Part model, mm, in its own coordinate system. Coordinates: 2 decimals unless noted, no trailing zeros. Write each loop counter-clockwise with the first axis right and the second up, starting at its lowest first coordinate (ties: lowest second). Pieces come first, ordered by that corner, then holes. Notation, with made-up numbers: (-18.5, -39) -> (-3.5, -39) arc R32 cw to (-3.5, -7) -> close; hole circle Ø7 at (-8, -22.5). An arc over 180 degrees is marked (long way). One line per question, with ' | ' between items. Start each with the question number.
Item 1: Saw through at B-B (y = -3.25). List the corners of the cut face in (x, z).
Item 2: Saw through at D-D (z = 0.25). List the corners of the cut face in (x, y), and give its area (3 significant figures).
Item 3: Saw through at C-C (x = 6). List the corners of the cut face in (y, z).
Item 4: Pin check, flat tips, straight feed: pin 1 (4 mm diameter, centred on x = -7, y = 4.5, fed in from -Z); pin 2 (1 mm diameter, centred on y = -5, z = 0.5, fed in from +X); pin 3 (1 mm diameter, centred on x = -6.5, z = 1, fed in from -Y). Stop position of each tip, or through.
Item 5: Probe probe 1 along Z at (x, y) = (-5, 4.5); probe 2 along Y at (x, z) = (1.5, 0.4); probe 3 along Y at (x, z) = (-3.25, 0.35). List the from-to ranges inside material, lowest first. Write a range as [from, to].
Item 6: Saw through at A-A (z = 1.75). List the corners of the cut face in (x, y).
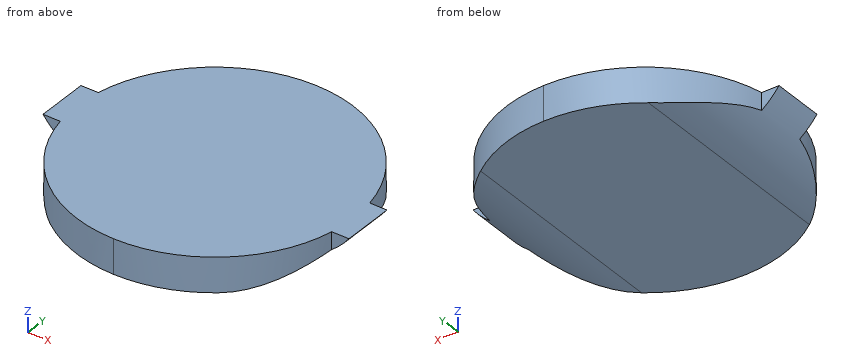
from build123d import *

# Parameters (mm, degrees)
F1_DEPTH    = 2
F2_T1_DEPTH = 23


# Not quite as in the source:
# - a fillet or chamfer that OpenCascade refuses, or shapes differently, is made with other operations: its cross-section is extruded or revolved along the edge and cut away or added


with BuildPart() as f1:
    # F0 (on Top) → F1 (new body)
    with BuildSketch(Plane.XY):
        with BuildLine():
            Line((0, 0), (8, 0))
            ThreePointArc((8, 0), (7.964450219, 0.7533476681), (7.8581168228, 1.5))
            ThreePointArc((7.8581168228, 1.5), (5.0990195136, 6.164414003), (0, 8))
            Line((0, 8), (0, 0))
        make_face()
        with BuildLine():
            Line((8.8581168228, 0), (8, 0))
            ThreePointArc((8, 0), (7.964450219, -0.7533476681), (7.8581168228, -1.5))
            Line((7.8581168228, -1.5), (8.8581168228, -1.5))
            Line((8.8581168228, -1.5), (8.8581168228, 0))
        make_face()
        with BuildLine():
            ThreePointArc((7.8581168228, 1.5), (7.964450219, 0.7533476681), (8, 0))
            Line((8, 0), (8.8581168228, 0))
            Line((8.8581168228, 0), (8.8581168228, 1.5))
            Line((8.8581168228, 1.5), (7.8581168228, 1.5))
        make_face()
        with BuildLine():
            ThreePointArc((7.8581168228, -1.5), (7.964450219, -0.7533476681), (8, 0))
            Line((8, 0), (0, 0))
            Line((0, 0), (0, -8))
            ThreePointArc((0, -8), (5.0990195136, -6.164414003), (7.8581168228, -1.5))
        make_face()
        with BuildLine():
            Line((-8, 0), (0, 0))
            Line((0, 0), (0, 8))
            ThreePointArc((0, 8), (-5.0990195136, 6.164414003), (-7.8581168228, 1.5))
            ThreePointArc((-7.8581168228, 1.5), (-7.964450219, 0.7533476681), (-8, 0))
        make_face()
        with BuildLine():
            Line((0, -8), (0, 0))
            Line((0, 0), (-8, 0))
            ThreePointArc((-8, 0), (-7.964450219, -0.7533476681), (-7.8581168228, -1.5))
            ThreePointArc((-7.8581168228, -1.5), (-5.0990195136, -6.164414003), (0, -8))
        make_face()
        with BuildLine():
            Line((-8.8581168228, 0), (-8, 0))
            ThreePointArc((-8, 0), (-7.964450219, 0.7533476681), (-7.8581168228, 1.5))
            Line((-7.8581168228, 1.5), (-8.8581168228, 1.5))
            Line((-8.8581168228, 1.5), (-8.8581168228, 0))
        make_face()
        with BuildLine():
            ThreePointArc((-7.8581168228, -1.5), (-7.964450219, -0.7533476681), (-8, 0))
            Line((-8, 0), (-8.8581168228, 0))
            Line((-8.8581168228, 0), (-8.8581168228, -1.5))
            Line((-8.8581168228, -1.5), (-7.8581168228, -1.5))
        make_face()
    extrude(amount=F1_DEPTH)

    # F2: fillet of radius 5 on 2 edges, made by hand

    # F2_s2 → F2_t1 (cut)
    with BuildSketch(Plane.XZ.offset(-11.5)):
        with BuildLine():
            ThreePointArc((-8.8581168228, 2), (-7.0941848003, 0.527864045), (-4.8581168228, 0))
            Line((-4.8581168228, 0), (-8.8581168228, 0))
            Line((-8.8581168228, 0), (-8.8581168228, 2))
        make_face()
        with BuildLine():
            ThreePointArc((8.8581168228, 2), (7.0941848003, 0.527864045), (4.8581168228, 0))
            Line((4.8581168228, 0), (8.8581168228, 0))
            Line((8.8581168228, 0), (8.8581168228, 2))
        make_face()
    extrude(amount=F2_T1_DEPTH, mode=Mode.SUBTRACT)


solid = f1.part
From the geometry:
1) outline: (-7.31, 0.64) arc R5 ccw to (-4.86, 0) -> (4.86, 0) arc R5 ccw to (7.31, 0.64) -> (7.31, 2) -> (-7.31, 2) -> close
2) outline: (-6.42, -4.77) arc R8 ccw to (6.42, -4.77) -> (6.42, 4.77) arc R8 ccw to (-6.42, 4.77) -> close | area: 181 mm2
3) outline: (-5.29, 0.13) -> (5.29, 0.13) -> (5.29, 2) -> (-5.29, 2) -> close
4) pin 1: z = 0 | pin 2: x = 6.61 | pin 3: y = -5.29
5) probe 1: [0, 2] | probe 2: [-7.86, 7.86] | probe 3: [-7.31, 7.31]
6) outline: (-8.66, -1.5) -> (-7.86, -1.5) arc R8 ccw to (7.86, -1.5) -> (8.66, -1.5) -> (8.66, 1.5) -> (7.86, 1.5) arc R8 ccw to (-7.86, 1.5) -> (-8.66, 1.5) -> close
